Geometry: final body of the model. Coordinates: model frame, mm. A direction names the side the tool comes from. Give positions to 0.01 mm unless a question says otherwise; leave off trailing zeros. Write each loop counter-clockwise with the first axis right and the second up, starting at its lowest first coordinate (ties: lowest second). Pieces come first, ordered by that corner, then holes. Notation, with made-up numbers: M -11.5,45.5 L 1.5,45.5 A20 cw 1.5,68.5 Z; hole C -8.75,34 d4. An arc over 180 degrees is marked long. Use a Markdown table: item, result. Add a question column.
1) Section C-C on z = 54. Return the cut outline in (x, y).
2) Pin query (flat end, axial travel): pin 1 (9 mm diameter, centred on y = -212.5, z = 37.5, fed in from +X); pin 2 (12 mm diameter, centred on y = -132.5, z = 22.5, fed in from -X); pin 3 (3 mm diameter, centred on x = 14, z = 59, fed in from -Y). Return the tip coordinate at first contact, or that it passes through.
3) Section B-B on y = -29. Return the cut outline in (x, z).
4) Draft query along Z for faces 1 (the flat face through (125, -126, 37)), 2 (the cylindrical face through (127.54, -239.31, 63.72)), 3 (the cylindrical face through (69.1, -2.5, 32)), 4 (the cylindrical face through (127.54, -239.31, 11.28)). Return one class per face: +Z half, -Z half, draft (parallel to the pull), parting line (faces both ways), or undercut.
5) Section D-D on x = 49. Return the cut outline in (y, z).
6) Set-up query: faces 5 (the flat face through (5, -129, 37)), 6 (the flat face through (2, -74, 75)). Return all of +Z, -Z, +X, -X, +Y, -Y with unobstructed straight access to the full face (end or side cutting, diameter ignored); none if empty.
7) Section A-A on x = 64. Return the cut outline in (y, z), then the cut area to 3 significant figures.
8) Line query: line 1 (Z direction, x = 1, y = -212); line 2 (X direction, y = -158, z = 60); line 3 (Y direction, x = 2, z = 37). Output: solid intervals per line, ascending.
```python
from build123d import *

# Parameters (mm, degrees)
BOSS_EXTRUDE1_DEPTH = 75
SKETCH2_R           = 7.5
CUT_EXTRUDE1_DEPTH  = 8
SKETCH3_R           = 5
CUT_EXTRUDE2_DEPTH  = 134
FILLET1_R           = 37.5


with BuildPart() as part:
    # Sketch1 → Boss-Extrude1 (new body)
    with BuildSketch(Plane.XY):
        Polygon((125, -250), (130, -250), (130, 0), (0, 0), (0, -250), (5, -250), (5, -5), (125, -5), align=None)
    extrude(amount=BOSS_EXTRUDE1_DEPTH)

    # Sketch2 → Cut-Extrude1 (cut)
    with BuildSketch(Plane(origin=(0, 0, 0), x_dir=(1, 0, 0), z_dir=(0, 1, 0))):
        with Locations(Location((64, -37.5, 0), (0, 0, 270))):
            Circle(SKETCH2_R)
    extrude(amount=-CUT_EXTRUDE1_DEPTH, mode=Mode.SUBTRACT)

    # Sketch3 → Cut-Extrude2 (cut)
    with BuildSketch(Plane(origin=(130, 0, 0), x_dir=(0, 0, -1), z_dir=(1, 0, 0))):
        with Locations(Location((-37.5, -212.5, 0), (0, 0, 90))):
            Circle(SKETCH3_R)
    extrude(amount=-CUT_EXTRUDE2_DEPTH, mode=Mode.SUBTRACT)

    # Fillet1
    fillet1_edges = [part.edges().sort_by_distance(p)[0] for p in [
        (127.5, -250, 75),
        (2.5, -250, 75),
        (2.5, -250, 0),
        (127.5, -250, 0),
    ]]
    fillet(fillet1_edges, radius=FILLET1_R - 0.0001)  # a hair under: the kernel refuses the full size


solid = part.part
```
Found:
| question | item | result |
|---|---|---|
| 1 | outline | M 0,-246.17 L 5,-246.17 L 5,-5 L 125,-5 L 125,-246.17 L 130,-246.17 L 130,0 L 0,0 Z |
| 2 | pin 1 | through |
| 2 | pin 2 | x = 0 |
| 2 | pin 3 | y = -5 |
| 3 | outline | M 0,0 L 5,0 L 5,75 L 0,75 Z; M 125,0 L 130,0 L 130,75 L 125,75 Z |
| 4 | face 1 | draft |
| 4 | face 2 | +Z half |
| 4 | face 3 | undercut |
| 4 | face 4 | -Z half |
| 5 | outline | M -5,0 L 0,0 L 0,75 L -5,75 Z |
| 6 | face 5 | +Z, -Z, -Y |
| 6 | face 6 | +Z, +X, -X, +Y, -Y |
| 7 | outline | M -5,0 L 0,0 L 0,30 L -5,30 Z; M -5,45 L 0,45 L 0,75 L -5,75 Z |
| 7 | area | 300 mm² |
| 8 | line 1 | 0 to 32.53, 42.47 to 75 |
| 8 | line 2 | 0 to 5, 125 to 130 |
| 8 | line 3 | -250 to -217.47, -207.53 to 0 |
